from build123d import *

# Parameters (mm, degrees)
SKETCH2_W           = 38.1
SKETCH2_H           = 254
BOSS_EXTRUDE1_DEPTH = 6.35
SIDE_EDGE_R         = 12.7
SIDE_EDGE_2_R       = 12.7
SKETCH4_R           = 3.175
SKETCH4_R_2         = 6.35
CUT_EXTRUDE1_DEPTH  = 257.920089717


with BuildPart() as part:
    # Sketch2 → Boss-Extrude1 (new body)
    with BuildSketch(Plane.XY):
        with Locations((19.05, 127)):
            Rectangle(SKETCH2_W, SKETCH2_H)
    extrude(amount=BOSS_EXTRUDE1_DEPTH)

    # Side Edge
    side_edge_edges = [part.edges().sort_by_distance(p)[0] for p in [
        (38.1, 254, 3.175),
    ]]
    fillet(side_edge_edges, radius=SIDE_EDGE_R)

    # Side Edge 2
    side_edge_2_edges = [part.edges().sort_by_distance(p)[0] for p in [
        (0, 254, 3.175),
    ]]
    fillet(side_edge_2_edges, radius=SIDE_EDGE_2_R)

    # Sketch4 → Cut-Extrude1 (cut, through all)
    with BuildSketch(Plane.XY.offset(6.35)):
        with Locations((29.21, 27.94)):
            Circle(SKETCH4_R)
        with Locations((29.21, 66.04)):
            Circle(SKETCH4_R)
        with Locations((19.812, 190.5)):
            Circle(SKETCH4_R_2)
    extrude(amount=-CUT_EXTRUDE1_DEPTH, mode=Mode.SUBTRACT)


solid = part.part
Input: part model. Units: mm. Frame: model coordinates. Round coordinates to 2 decimals unless told otherwise and drop trailing zeros. Write each loop counter-clockwise with the first axis right and the second up, starting at its lowest first coordinate (ties: lowest second). Pieces come first, ordered by that corner, then holes.
1) Cut plane C-C (z = 4). Return the cut outline in (x, y) (3 decimals), then the cut area to 3 significant figures.
2) Cut plane A-A (y = 27.94). Return the cut outline in (x, z) (3 decimals), then the cut area to 3 significant figures.
3) Cut plane D-D (x = 29.21). Return the cut outline in (y, z) (3 decimals).
4) Ray query, L1, parallel to Y at x = 29.21, z = 2 (3 decimals); L2, parallel to Y at x = 25, z = 5.5; L3, parallel to Y at x = 23, z = 5. Return the intervals inside material, ascending.
5) Contact query for a flat-ended pin moving along its axis: P1, Ø5.5, axis at x = 29.21, y = 27.94, coming from the +Z side. Output: stop coordinate, or through.
6) Draft query along Y for faces 1 (the cylindrical face through (34.48, 250.18, 3.22)), 2 (the flat face through (19, 129, 6.35)), 3 (the cylindrical face through (18.985, 196.796, 3.219)), 4 (the cylindrical face through (30.675, 25.123, 3.219)). Return one class per face: pulls with the +Y half, pulls with the -Y half, needs draft (parallel to the pull), parting line crosses it, or undercut.
7) Cut plane B-B (x = 18). Return the cut outline in (y, z).
Geometry says:
1. outline: (0, 0) - (38.1, 0) - (38.1, 241.3) arc R12.7 ccw to (25.4, 254) - (12.7, 254) arc R12.7 ccw to (0, 241.3) - close; hole circle Ø12.7 at (19.812, 190.5); hole circle Ø6.35 at (29.21, 27.94); hole circle Ø6.35 at (29.21, 66.04)
1. area: 9,420 mm2
2. outline: (0, 0) - (26.035, 0) - (26.035, 6.35) - (0, 6.35) - close; (32.385, 0) - (38.1, 0) - (38.1, 6.35) - (32.385, 6.35) - close
2. area: 202 mm2
3. outline: (0, 0) - (24.765, 0) - (24.765, 6.35) - (0, 6.35) - close; (31.115, 0) - (62.865, 0) - (62.865, 6.35) - (31.115, 6.35) - close; (69.215, 0) - (253.415, 0) - (253.415, 6.35) - (69.215, 6.35) - close
4. L1: y = 0 to 24.765, 31.115 to 62.865, 69.215 to 253.415
4. L2: y = 0 to 186.84, 194.16 to 254
4. L3: y = 0 to 185.01, 195.99 to 254
5. P1: passes through
6. face 1: pulls with the +Y half
6. face 2: needs draft
6. face 3: undercut
6. face 4: undercut
7. outline: (0, 0) - (184.41, 0) - (184.41, 6.35) - (0, 6.35) - close; (196.59, 0) - (254, 0) - (254, 6.35) - (196.59, 6.35) - close
